Here's how the part is built. I have some questions about the finished solid (model axes, mm). A direction names the side the tool comes from. Round coordinates to 2 decimals unless told otherwise and drop trailing zeros. Order: outer loops, then holes, each group sorted by start corner. A loop starts at its lowest first (then second) coordinate and runs counter-clockwise, first axis right, second up.
```python
from build123d import *

# Parameters (mm, degrees)
SKETCH1_W                        = 25.4
SKETCH1_H                        = 50.8
SKETCH1_W_2                      = 19.05
SKETCH1_H_2                      = 44.45
BOSS_EXTRUDE1_DEPTH              = 825.5
SKETCH2_R                        = 14.2875
CUT_EXTRUDE1_DEPTH               = 828.451539367
SKETCH3_R                        = 2.5796875
CUT_EXTRUDE2_DEPTH               = 828.451539367
F_13_64_0_20313_DIAMETER_HOLE1_D = 5.159502
SKETCH6_R                        = 3.3734375
SKETCH6_R_2                      = 3.429
CUT_EXTRUDE3_DEPTH               = 828.451539367
CUT_EXTRUDE4_DEPTH               = 828.451539367
LPATTERN1_COUNT                  = 9
LPATTERN1_PITCH                  = 59.69


with BuildPart() as part:
    # Sketch1 → Boss-Extrude1 (new body)
    with BuildSketch(Plane(origin=(0, 0, 0), x_dir=(1, 0, 0), z_dir=(0, 1, 0))):
        with Locations((12.7, 25.4)):
            Rectangle(SKETCH1_W, SKETCH1_H)
        with Locations((12.7, 25.4)):
            Rectangle(SKETCH1_W_2, SKETCH1_H_2, mode=Mode.SUBTRACT)
    extrude(amount=BOSS_EXTRUDE1_DEPTH)

    # Sketch2 → Cut-Extrude1 (cut, through all)
    with BuildSketch(Plane.ZY):
        with Locations((-25.4, 38.1)):
            Circle(SKETCH2_R)
    extrude(amount=-CUT_EXTRUDE1_DEPTH, mode=Mode.SUBTRACT)

    # Sketch3 → Cut-Extrude2 (cut, through all)
    with BuildSketch(Plane.XY):
        with Locations((12.7, 812.8)):
            Circle(SKETCH3_R)
        with Locations((12.7, 762)):
            Circle(SKETCH3_R)
    extrude(amount=-CUT_EXTRUDE2_DEPTH, mode=Mode.SUBTRACT)

    # 13/64 (0.20313) Diameter Hole1 (through all)
    with Locations(Plane(origin=(25.4, 0, 0), x_dir=(0, 0, -1), z_dir=(1, 0, 0))):
        with Locations((37.30625, 58.722229928), (13.49375, 58.722229928), (37.30625, 17.477770072), (13.49375, 17.477770072)):
            Hole(F_13_64_0_20313_DIAMETER_HOLE1_D / 2)

    # Sketch6 → Cut-Extrude3 (cut, through all)
    with BuildSketch(Plane(origin=(0, 0, -50.8), x_dir=(-1, 0, 0), z_dir=(0, 0, -1))):
        with Locations((-12.7, 353.06)):
            Circle(SKETCH6_R)
        with Locations((-12.7, 289.56)):
            Circle(SKETCH6_R_2)
    extrude(amount=-CUT_EXTRUDE3_DEPTH, mode=Mode.SUBTRACT)

    # Sketch7 → Cut-Extrude4 (cut, through all)
    with BuildSketch(Plane(origin=(25.4, 0, 0), x_dir=(0, 0, -1), z_dir=(1, 0, 0))):
        Polygon((41.91, 273.064105889), (8.89, 292.128211777), (8.89, 254), align=None)
        Polygon((41.91, 321.457605452), (8.89, 302.393499563), (41.91, 283.329393675), align=None)
    cut_extrude4 = extrude(amount=-CUT_EXTRUDE4_DEPTH, mode=Mode.SUBTRACT)

    # LPattern1: Cut-Extrude4 ×9
    with Locations(*[(0, i * LPATTERN1_PITCH, 0) for i in range(1, LPATTERN1_COUNT)]):
        add(cut_extrude4, mode=Mode.SUBTRACT)


solid = part.part
```
1. On a 3-axis mill with a long thin cutter (end or side, diameter ignored), from which of +Z, -Z, +X, -X, +Y, -Y can I reach the whole of each face in a straight line? I mean faces 4 (the flat face through (23.835, 461.533, -25.631)), 5 (the flat face through (13, 407, -3.175)). Say none if no direction works.
Evaluation:
face 4: +X, -X
face 5: +Y, -Y
2. If we section it at A-A, the plane y = 38.1: Write out the boundary of the cut face in (x, z) (1 decimal), and give its area (3 significant figures).
Evaluation:
outline: (0, -50.8) - (25.4, -50.8) - (25.4, -39.7) - (22.2, -39.7) - (22.2, -47.6) - (3.2, -47.6) - (3.2, -39.7) - (0, -39.7) - close; (0, -11.1) - (3.2, -11.1) - (3.2, -3.2) - (22.2, -3.2) - (22.2, -11.1) - (25.4, -11.1) - (25.4, 0) - (0, 0) - close
area: 262 mm2
3. I need wall thicknesses on probe 1 along Y at (x, z) = (12.7, -49.05); probe 2 along X at (y, z) = (375, -5) (3 decimals); probe 3 along Z at (x, y) = (8.25, 189.5) (3 decimals). Which ranges of each line are inside material? Lowest first, please.
Evaluation:
probe 1: y = 0 to 286.13, 292.99 to 349.69, 356.43 to 759.42, 764.58 to 810.22, 815.38 to 825.5
probe 2: x = 0 to 3.175, 22.225 to 25.4
probe 3: z = -50.8 to -47.625, -3.175 to 0
4. If we section it at B-B, the plane z = -23: State how many separate pieces and enclosed holes the cut face has, and give its area (3 significant figures).
Evaluation:
separate pieces: 40
enclosed holes: 0
area: 2,880 mm2
5. If we mould it in two halves opening along Z, with no side actions, what happens to faces 1 (the flat face through (1.61, 651.135, -25.169)), 2 (the flat face through (13, 407, 0)), 3 (the flat face through (2, 0, -24))? For each: released by +Z, released by -Z, zero draft, split by the parting line, or undercut.
Evaluation:
face 1: undercut
face 2: released by +Z
face 3: zero draft
